The listing builds one solid part. Answer for the finished solid, in the listing's coordinates (mm). Face numbers are marked on the shaded views. A direction names the side the tool comes from. Give positions to 0.01 mm unless a question says otherwise; leave off trailing zeros. Write each loop counter-clockwise with the first axis right and the second up, starting at its lowest first coordinate (ties: lowest second). Pieces come first, ordered by that corner, then holes. Notation, with made-up numbers: (56, 66.25) -> (88, 66.25) arc R30 cw to (88, 103.25) -> close; hole circle Ø4 at (65.25, -26.75). An arc over 180 degrees is marked (long way). Use CSV: the item, a comma, the result in double quotes. Start each with the question number.
from build123d import *

# Parameters (mm, degrees)
F0_W     = 150
F0_H     = 63.5
F1_DEPTH = 5
F3_DEPTH = 10.001
F5_D     = 9
F5_DEPTH = 18
F5_TIP   = 2.7038727856


with BuildPart() as f1:
    # F0 (on Front) → F1 (new body, symmetric)
    with BuildSketch(Plane.XZ):
        Rectangle(F0_W, F0_H)
    extrude(amount=F1_DEPTH, both=True)

    # F2 (on face) → F3 (cut, through all)
    with BuildSketch(Plane.XZ.offset(5)):
        with BuildLine():
            ThreePointArc((-60, 19.5), (-64.5, 15), (-60, 10.5))
            Line((-60, 10.5), (-10, 10.5))
            ThreePointArc((-10, 10.5), (-5.5, 15), (-10, 19.5))
            Line((-10, 19.5), (-60, 19.5))
        make_face()
        with BuildLine():
            ThreePointArc((-60, -10.5), (-64.5, -15), (-60, -19.5))
            Line((-60, -19.5), (-10, -19.5))
            ThreePointArc((-10, -19.5), (-5.5, -15), (-10, -10.5))
            Line((-10, -10.5), (-60, -10.5))
        make_face()
    extrude(amount=-F3_DEPTH, mode=Mode.SUBTRACT)

    # F5
    with Locations(Plane.XZ.offset(5)):
        with Locations((35, 0), (63.6, 20.65), (63.6, -20.65)):
            Hole(F5_D / 2, depth=F5_DEPTH)
            with Locations((0, 0, -(F5_DEPTH + F5_TIP / 2))):  # 118° drill point
                Cone(0, F5_D / 2, F5_TIP, mode=Mode.SUBTRACT)


solid = f1.part
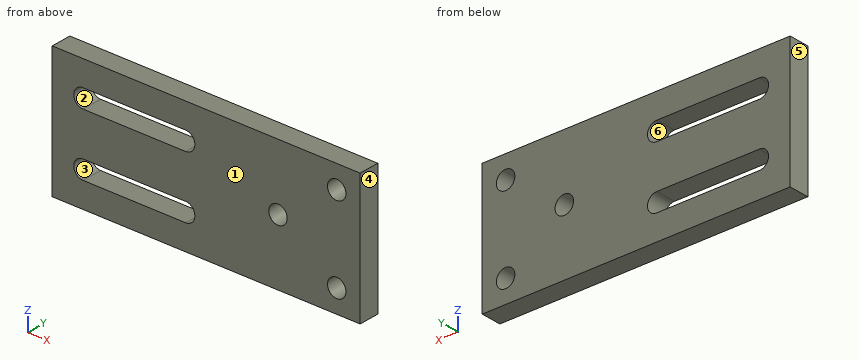
Q1. The mould has two halves that part along X. Classify the marked faces 1, 2, 3 and 4: +X half, -X half, draft (parallel to the pull), parting line (faces both ways), or undercut.
Q2. Section A-A on x = 35 is taken. Give the vertices of the cut face in (y, z), then the cut area to 3 significant figures.
Q3. A flat-ended cylindrical pin translates along its axis: pin 1 Ø8 at (x, z) = (63.6, -20.65) entering from -Y. Find the tip coordinate at first contact, or state that the pin passes through.
Q4. For the marked faces 5 and 6, determine the directions among +Z, -Z, +X, -X, +Y, -Y from which every point of the face is accessible in a straight line to the end or side of a thin tool.
Q5. Section C-C on x = -45 is taken. Give the vertices of the cut face in (y, z).
Q6. Straight lines are drawn through the part: L1, parallel to Z at x = -60.5, y = -4.25; L2, parallel to Z at x = 63.6, y = 1.5; L3, parallel to X at y = -0.25, z = -16.5. For each, find the intervals that lie inside material, in ascending order.
Q7. Section B-B on y = -2.25 is taken. Give the vertices of the cut face in (x, z), then the cut area to 3 significant figures.
Output:
1,face 1,"draft"
1,face 2,"undercut"
1,face 3,"undercut"
1,face 4,"+X half"
2,outline,"(-5, -31.75) -> (5, -31.75) -> (5, -4.5) -> (-5, -4.5) -> close; (-5, 4.5) -> (5, 4.5) -> (5, 31.75) -> (-5, 31.75) -> close"
2,area,"545 mm²"
3,pin 1,"through"
4,face 5,"+Z, -Z, -X, +Y, -Y"
4,face 6,"+Y, -Y"
5,outline,"(-5, -31.75) -> (5, -31.75) -> (5, -19.5) -> (-5, -19.5) -> close; (-5, -10.5) -> (5, -10.5) -> (5, 10.5) -> (-5, 10.5) -> close; (-5, 19.5) -> (5, 19.5) -> (5, 31.75) -> (-5, 31.75) -> close"
6,L1,"-31.75 to -19.47, -10.53 to 10.53, 19.47 to 31.75"
6,L2,"-31.75 to -25.15, -16.15 to 16.15, 25.15 to 31.75"
6,L3,"-75 to -64.24, -5.76 to 61.86, 65.34 to 75"
7,outline,"(-75, -31.75) -> (75, -31.75) -> (75, 31.75) -> (-75, 31.75) -> close; hole (-60, -19.5) -> (-10, -19.5) arc R4.5 ccw to (-10, -10.5) -> (-60, -10.5) arc R4.5 ccw to start; hole (-60, 10.5) -> (-10, 10.5) arc R4.5 ccw to (-10, 19.5) -> (-60, 19.5) arc R4.5 ccw to start; hole circle Ø9 at (35, 0); hole circle Ø9 at (63.6, -20.65); hole circle Ø9 at (63.6, 20.65)"
7,area,"8,310 mm²"
